```python
from build123d import *

# Parameters (mm, degrees)
SKETCH1_W                 = 20
SKETCH1_H                 = 82.5
BOSS_EXTRUDE1_DEPTH       = 600
SKETCH2_R                 = 1.35
CUT_EXTRUDE1_DEPTH        = 600
CUT_EXTRUDE4_DEPTH        = 600
SKETCH6_W                 = 16.969486996
SKETCH6_H                 = 44.5
CUT_EXTRUDE5_DEPTH        = 600
F_4_0MM_DOWEL_HOLE3_D     = 4
F_4_0MM_DOWEL_HOLE3_DEPTH = 14
F_4_0MM_DOWEL_HOLE3_TIP   = 1.201721238
F_4_0MM_DOWEL_HOLE2_D     = 4
F_4_0MM_DOWEL_HOLE2_DEPTH = 14
F_4_0MM_DOWEL_HOLE2_TIP   = 1.201721238
F_4_0MM_DOWEL_HOLE4_D     = 4
F_4_0MM_DOWEL_HOLE4_DEPTH = 14
F_4_0MM_DOWEL_HOLE4_TIP   = 1.201721238
F_4_0MM_DOWEL_HOLE5_D     = 4
F_4_0MM_DOWEL_HOLE5_DEPTH = 14
F_4_0MM_DOWEL_HOLE5_TIP   = 1.201721238


with BuildPart() as part:
    # Sketch1 → Boss-Extrude1 (new body)
    with BuildSketch(Plane.XY):
        with Locations((5.517241379, -30.301724138)):
            Rectangle(SKETCH1_W, SKETCH1_H)
    extrude(amount=BOSS_EXTRUDE1_DEPTH)

    # Sketch2 → Cut-Extrude1 (cut)
    with BuildSketch(Plane(origin=(0, 10.948275862, 0), x_dir=(1, 0, 0), z_dir=(0, 1, 0))):
        with Locations(Location((9.329077472, -3.272098327, 0), (0, 0, 270))):
            Circle(SKETCH2_R)
        with Locations(Location((1.705405286, -7.303246399, 0), (0, 0, 270))):
            Circle(SKETCH2_R)
    extrude(amount=-CUT_EXTRUDE1_DEPTH, mode=Mode.SUBTRACT)

    # Sketch5 → Cut-Extrude4 (cut)
    with BuildSketch(Plane.ZY.offset(4.482758621)):
        Polygon((40, -51.551724138), (600, -51.551724138), (600, 10.948275862), (16.969486996, 10.948275862), align=None)
    extrude(amount=-CUT_EXTRUDE4_DEPTH, mode=Mode.SUBTRACT)

    # Sketch6 → Cut-Extrude5 (cut)
    with BuildSketch(Plane.ZY.offset(4.482758621)):
        with Locations((8.484743498, -49.301724138)):
            Rectangle(SKETCH6_W, SKETCH6_H)
    extrude(amount=-CUT_EXTRUDE5_DEPTH, mode=Mode.SUBTRACT)

    # Ø4.0mm Dowel Hole3
    with Locations(Plane.XZ.offset(71.551724138)):
        with Locations((10.517241379, 84.246230703), (10.517241379, 99.246230703), (10.517241379, 224.909334592), (10.517241379, 239.909334592), (10.517241379, 535), (10.517241379, 550)):
            Hole(F_4_0MM_DOWEL_HOLE3_D / 2, depth=F_4_0MM_DOWEL_HOLE3_DEPTH)
            with Locations((0, 0, -(F_4_0MM_DOWEL_HOLE3_DEPTH + F_4_0MM_DOWEL_HOLE3_TIP / 2))):  # 118° drill point
                Cone(0, F_4_0MM_DOWEL_HOLE3_D / 2, F_4_0MM_DOWEL_HOLE3_TIP, mode=Mode.SUBTRACT)

    # Ø4.0mm Dowel Hole2
    with Locations(Plane.XZ.offset(71.551724138)):
        with Locations((0.517241379, 550), (0.517241379, 535)):
            Hole(F_4_0MM_DOWEL_HOLE2_D / 2, depth=F_4_0MM_DOWEL_HOLE2_DEPTH)
            with Locations((0, 0, -(F_4_0MM_DOWEL_HOLE2_DEPTH + F_4_0MM_DOWEL_HOLE2_TIP / 2))):  # 118° drill point
                Cone(0, F_4_0MM_DOWEL_HOLE2_D / 2, F_4_0MM_DOWEL_HOLE2_TIP, mode=Mode.SUBTRACT)

    # Ø4.0mm Dowel Hole4
    with Locations(Plane.XZ.offset(71.551724138)):
        with Locations((0.517241379, 99.246230703), (0.517241379, 84.246230703)):
            Hole(F_4_0MM_DOWEL_HOLE4_D / 2, depth=F_4_0MM_DOWEL_HOLE4_DEPTH)
            with Locations((0, 0, -(F_4_0MM_DOWEL_HOLE4_DEPTH + F_4_0MM_DOWEL_HOLE4_TIP / 2))):  # 118° drill point
                Cone(0, F_4_0MM_DOWEL_HOLE4_D / 2, F_4_0MM_DOWEL_HOLE4_TIP, mode=Mode.SUBTRACT)

    # Ø4.0mm Dowel Hole5
    with Locations(Plane.XZ.offset(71.551724138)):
        with Locations((0, 224.909334592), (0, 239.909334592)):
            Hole(F_4_0MM_DOWEL_HOLE5_D / 2, depth=F_4_0MM_DOWEL_HOLE5_DEPTH)
            with Locations((0, 0, -(F_4_0MM_DOWEL_HOLE5_DEPTH + F_4_0MM_DOWEL_HOLE5_TIP / 2))):  # 118° drill point
                Cone(0, F_4_0MM_DOWEL_HOLE5_D / 2, F_4_0MM_DOWEL_HOLE5_TIP, mode=Mode.SUBTRACT)


solid = part.part
```
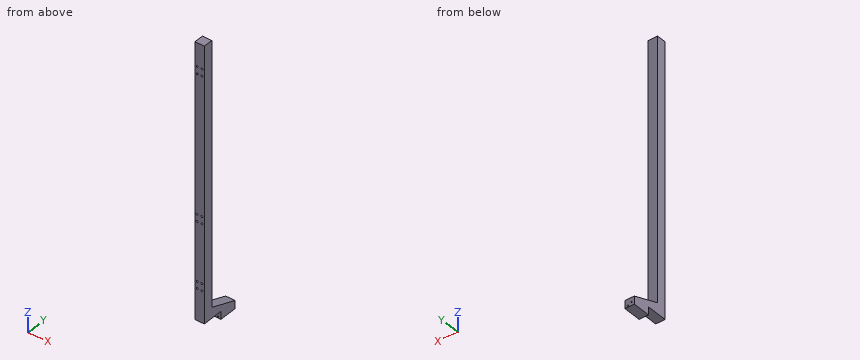
Model file for the job. Use its own axes, mm. Coordinates: 2 decimals unless noted, no trailing zeros. Order: outer loops, then holes, each group sorted by start corner. A loop starts at its lowest first (then second) coordinate and runs counter-clockwise, first axis right, second up. Notation, with made-up numbers: (-18.75, 69.25) - (-12.75, 69.25) arc R9 ccw to (-12.75, 76.25) - close; hole circle Ø5 at (-33.5, 65). An arc over 180 degrees is marked (long way). Return JSON: item names as keys, results as strings. Group by question number.
1) Probe line 1 (X direction, y = -67, z = 535); line 2 (Y direction, x = -2, z = 82.5); line 3 (Z direction, x = 13.5, y = -67). List the from-to ranges inside material, lowest first. Write a range as from..to.
2) Saw through at A-A, the plane y = -22. Write the cut outline in (x, z), plus the area to 3 significant figures.
3) Saw through at C-C, the plane y = -43.5. Write the cut outline in (x, z).
4) Flat gauge pins, fed straight in: P1, Ø10, axis at x = 7, y = -34, coming from the -Z side; P2, Ø3, axis at x = 0.52, z = 550, coming from the +Y side; P3, Ø3, axis at x = 10.52, z = 239.91, coming from the -Y side. Where does each tip first touch, or does it go through?
5) Saw through at B-B, the plane z = 277. Write the cut outline in (x, y), plus the area to 3 significant figures.
Values found:
{
 "1": {"line 1": "x = -4.48..-1.48, 2.52..8.52, 12.52..15.52", "line 2": "y = -71.55..-51.55", "line 3": "z = 16.97..600"},
 "2": {"outline": "(-4.48, 0) - (15.52, 0) - (15.52, 29.11) - (-4.48, 29.11) - close; hole circle Ø2.7 at (1.71, 7.3); hole circle Ø2.7 at (9.33, 3.27)", "area": "571 mm²"},
 "3": {"outline": "(-4.48, 16.97) - (15.52, 16.97) - (15.52, 37.03) - (-4.48, 37.03) - close"},
 "4": {"P1": "stops at z = 16.97", "P2": "stops at y = -51.55", "P3": "stops at y = -57.25"},
 "5": {"outline": "(-4.48, -71.55) - (15.52, -71.55) - (15.52, -51.55) - (-4.48, -51.55) - close", "area": "400 mm²"}
}
